```python
from build123d import *
from build123d.topology import SkipClean

# Parameters (mm, degrees)
SKETCH_2_W           = 5
SKETCH_2_H           = 10
EXTRUDE_1_DEPTH      = 0.5
CUT_EXTRUDE_1_DEPTH  = 1.5
EXTRUDE_3_DEPTH      = 0.5
SKETCH_8_R           = 0.6
CUT_EXTRUDE_2_DEPTH  = 0.5
SKETCH_12_W          = 5
SKETCH_12_H          = 0.5
EXTRUDE_4_DEPTH      = 10.5
SKETCH_14_W          = 5
SKETCH_14_H          = 0.5
EXTRUDE_5_DEPTH      = 10
SKETCH_16_W          = 5
SKETCH_16_H          = 0.5
CUT_EXTRUDE_3_DEPTH  = 10
CUT_EXTRUDE_4_DEPTH  = 10
EXTRUDE_START        = -0.5
EXTRUDE_6_DEPTH      = 0.5
SKETCH_19_R          = 0.6
CUT_EXTRUDE_5_DEPTH  = 0.5
SKETCH_23_W          = 0.5
SKETCH_23_H          = 1.5
EXTRUDE_7_DEPTH      = 0.5
EXTRUDE_9_DEPTH      = 0.5
SKETCH_25_R          = 0.25
CUT_EXTRUDE_6_DEPTH  = 0.5
CUT_EXTRUDE_START    = -0.5
SKETCH_28_R          = 0.25
CUT_EXTRUDE_7_DEPTH  = 0.5
SCALE_1_SCALE        = 3.181818182
SCALE_2_SCALE        = 0.771428571
CUT_EXTRUDE_8_DEPTH  = 10
SKETCH_30_R          = 1.75
CUT_EXTRUDE_9_DEPTH  = 10
EXTRUDE_10_DEPTH     = 3
SKETCH_37_R          = 4.295454545
EXTRUDE_11_DEPTH     = 3
CUT_EXTRUDE_START_2  = -3
SKETCH_38_R          = 1.75
CUT_EXTRUDE_10_DEPTH = 3
SKETCH_39_R          = 1.75
CUT_EXTRUDE_11_DEPTH = 3
SKETCH_41_W          = 46.80206249
SKETCH_41_H          = 2.589600393
CUT_EXTRUDE_13_DEPTH = 30.175477213
SKETCH_42_W          = 32.065343688
SKETCH_42_H          = 1.095167369
CUT_EXTRUDE_14_DEPTH = 30.175477212
EXTRUDE_START_2      = 0.77
EXTRUDE_12_DEPTH     = 0.77
CUT_EXTRUDE_15_REACH = 34.524
SKETCH_44_R          = 1.75


with BuildPart() as part:
    # 草图2 → 凸台-拉伸1 (new body)
    with BuildSketch(Plane(origin=(0, 0, 0), x_dir=(1, 0, 0), z_dir=(0, 1, 0))):
        Rectangle(SKETCH_2_W, SKETCH_2_H)
    extrude(amount=EXTRUDE_1_DEPTH)

    # 草图3 → 切除-拉伸1 (cut)
    with BuildSketch(Plane(origin=(0, 0.5, 0), x_dir=(1, 0, 0), z_dir=(0, 1, 0))):
        Polygon((-2.5, 0), (-1, 5), (-4.597388324, 7.155522044), (-6.097388324, 2.155522044), align=None)
    extrude(amount=-CUT_EXTRUDE_1_DEPTH, mode=Mode.SUBTRACT)

    # 草图6 → 凸台-拉伸3 (add)
    with BuildSketch(Plane.XZ):
        with BuildLine():
            Line((-1, -5), (2.5, -5))
            ThreePointArc((2.5, -5), (0.75, -6.75), (-1, -5))
        make_face()
    extrude(amount=-EXTRUDE_3_DEPTH)

    # 草图8 → 切除-拉伸2 (cut)
    with BuildSketch(Plane(origin=(0, 0.5, 0), x_dir=(1, 0, 0), z_dir=(0, 1, 0))):
        with Locations(Location((0.858368729, 4.996789463, 0), (0, 0, 270))):
            Circle(SKETCH_8_R)
    extrude(amount=-CUT_EXTRUDE_2_DEPTH, mode=Mode.SUBTRACT)

    # 草图12 → 凸台-拉伸4 (add)
    with BuildSketch(Plane.XZ):
        with Locations((0, 4.75)):
            Rectangle(SKETCH_12_W, SKETCH_12_H)
    extrude(amount=EXTRUDE_4_DEPTH)

    # 草图14 → 凸台-拉伸5 (add)
    with BuildSketch(Plane(origin=(0, 0, 4.5), x_dir=(-1, 0, 0), z_dir=(0, 0, -1))):
        with Locations((0, -10.25)):
            Rectangle(SKETCH_14_W, SKETCH_14_H)
    extrude(amount=EXTRUDE_5_DEPTH)

    # 草图16 → 切除-拉伸3 (cut)
    with BuildSketch(Plane(origin=(0, -10, 0), x_dir=(1, 0, 0), z_dir=(0, 1, 0))):
        with Locations((0, 5.25)):
            Rectangle(SKETCH_16_W, SKETCH_16_H)
    extrude(amount=-CUT_EXTRUDE_3_DEPTH, mode=Mode.SUBTRACT)

    # 草图17 → 切除-拉伸4 (cut)
    with BuildSketch(Plane(origin=(0, -10, 0), x_dir=(1, 0, 0), z_dir=(0, 1, 0))):
        Polygon((-1, 5), (-2.5, 0), (-4.860653069, 1.950314005), (-3.360653069, 6.950314005), align=None)
    extrude(amount=-CUT_EXTRUDE_4_DEPTH, mode=Mode.SUBTRACT)

    # 草图18 → 凸台-拉伸6 (add)
    with BuildSketch(Plane(origin=(0, -10, 0), x_dir=(1, 0, 0), z_dir=(0, 1, 0)).offset(EXTRUDE_START)):
        with BuildLine():
            Line((-1, 5), (2.5, 5))
            ThreePointArc((2.5, 5), (0.75, 6.75), (-1, 5))
        make_face()
    extrude(amount=EXTRUDE_6_DEPTH)

    # 草图19 → 切除-拉伸5 (cut)
    with BuildSketch(Plane(origin=(0, -10, 0), x_dir=(1, 0, 0), z_dir=(0, 1, 0))):
        with Locations(Location((0.858368729, 4.996789463, 0), (0, 0, 270))):
            Circle(SKETCH_19_R)
    extrude(amount=-CUT_EXTRUDE_5_DEPTH, mode=Mode.SUBTRACT)

    # 草图23 → 凸台-拉伸7 (add)
    with BuildSketch(Plane.XY.offset(5)):
        with Locations((2.25, -0.25)):
            Rectangle(SKETCH_23_W, SKETCH_23_H)
    extrude_7 = extrude(amount=EXTRUDE_7_DEPTH)

    # 草图24 → 凸台-拉伸9 (add)
    with BuildSketch(Plane(origin=(2.5, 0, 0), x_dir=(0, 0, -1), z_dir=(1, 0, 0))):
        with BuildLine():
            Line((-5.5, 0.5), (-5.5, -1))
            ThreePointArc((-5.5, -1), (-6.25, -0.25), (-5.5, 0.5))
        make_face()
    extrude_9 = extrude(amount=-EXTRUDE_9_DEPTH)

    # 草图25 → 切除-拉伸6 (cut)
    with BuildSketch(Plane(origin=(2.5, 0, 0), x_dir=(0, 0, -1), z_dir=(1, 0, 0))):
        with Locations((-5.5, -0.25)):
            Circle(SKETCH_25_R)
    extrude(amount=-CUT_EXTRUDE_6_DEPTH, mode=Mode.SUBTRACT)

    # 镜向1: 凸台-拉伸7, 凸台-拉伸9 across plane
    add(extrude_7.mirror(Plane(origin=(0, 0, 0), x_dir=(0, 0, 1), z_dir=(1, 0, 0))))
    add(extrude_9.mirror(Plane(origin=(0, 0, 0), x_dir=(0, 0, 1), z_dir=(1, 0, 0))))

    # 草图28 → 切除-拉伸7 (cut)
    with BuildSketch(Plane.ZY.offset(2.5).offset(CUT_EXTRUDE_START)):
        with Locations(Location((5.5, -0.25, 0), (0, 0, 180))):
            Circle(SKETCH_28_R)
    extrude(amount=CUT_EXTRUDE_7_DEPTH, mode=Mode.SUBTRACT)


with BuildPart() as part_1:
    # 缩放比例1: scaled about (0.132742616, -4.910605003, 1.535666779)
    add(part.part.scale(SCALE_1_SCALE).moved(Location((-0.289620253, 10.714047279, -3.3505457))))


with BuildPart() as part_2:
    # 缩放比例2: scaled about (0.132742617, -4.910605002, 1.53566678)
    add(part_1.part.scale(SCALE_2_SCALE).moved(Location((0.03034117, -1.122424, 0.35100955))))

    # 草图29 → 切除-拉伸8 (cut)
    with BuildSketch(Plane(origin=(0, 8.369970913, 0), x_dir=(1, 0, 0), z_dir=(0, 1, 0))):
        with BuildLine():
            ThreePointArc((3.397828922, 14.506424406), (1.647828922, 16.256424406), (-0.102171078, 14.506424406))
            Line((-0.102171078, 14.506424406), (0.441118704, 14.506424406))
            ThreePointArc((0.441118704, 14.506424406), (1.913824893, 15.97127127), (3.386531082, 14.506424406))
            Line((3.386531082, 14.506424406), (3.397828922, 14.506424406))
        make_face()
        with BuildLine():
            Line((0.441118704, 14.506424406), (-0.102171078, 14.506424406))
            ThreePointArc((-0.102171078, 14.506424406), (1.647828922, 12.756424406), (3.397828922, 14.506424406))
            Line((3.397828922, 14.506424406), (3.386531082, 14.506424406))
            ThreePointArc((3.386531082, 14.506424406), (3.386546895, 14.502484216), (3.386552166, 14.498543997))
            ThreePointArc((3.386552166, 14.498543997), (1.909884674, 13.025821995), (0.441118704, 14.506424406))
        make_face()
    extrude(amount=-CUT_EXTRUDE_8_DEPTH, mode=Mode.SUBTRACT)

    # 草图30 → 切除-拉伸9 (cut)
    with BuildSketch(Plane(origin=(0, 8.369970913, 0), x_dir=(1, 0, 0), z_dir=(0, 1, 0))):
        with Locations(Location((1.511995488, 4.506424406, 0), (0, 0, 270))):
            Circle(SKETCH_30_R)
    extrude(amount=-CUT_EXTRUDE_9_DEPTH, mode=Mode.SUBTRACT)

    # 草图33 → 凸台-拉伸10 (add)
    with BuildSketch(Plane(origin=(0, 8.369970913, 0), x_dir=(1, 0, 0), z_dir=(0, 1, 0))):
        Polygon((-5.102171078, -10.039030139), (-5.102171078, -11.266302866), (-6.329443805, -11.266302866), (-6.329443805, 2.233697134), (-2.647625624, 14.506424406), (5.943283467, 14.506424406), (5.943283467, -11.266302866), (4.71601074, -11.266302866), (4.71601074, -10.039030139), align=None)
    extrude(amount=EXTRUDE_10_DEPTH)

    # 草图37 → 凸台-拉伸11 (add)
    with BuildSketch(Plane(origin=(0, 8.369970913, 0), x_dir=(1, 0, 0), z_dir=(0, 1, 0))):
        with Locations((1.647828922, 14.506424406)):
            Circle(SKETCH_37_R)
    extrude(amount=EXTRUDE_11_DEPTH)

    # 草图38 → 切除-拉伸10 (cut)
    with SkipClean():  # the faces are left unmerged after this step: merging them gives an invalid solid
        with BuildSketch(Plane(origin=(0, 8.369970913, 0), x_dir=(-1, 0, 0), z_dir=(0, -1, 0)).offset(CUT_EXTRUDE_START_2)):
            with Locations(Location((-1.647828922, 14.506424406, 0), (0, 0, 270))):
                Circle(SKETCH_38_R)
        extrude(amount=CUT_EXTRUDE_10_DEPTH, mode=Mode.SUBTRACT)

    # 草图39 → 切除-拉伸11 (cut)
    with BuildSketch(Plane(origin=(0, 8.369970913, 0), x_dir=(-1, 0, 0), z_dir=(0, -1, 0)).offset(CUT_EXTRUDE_START_2)):
        with Locations(Location((-1.511995488, 4.506424406, 0), (0, 0, 270))):
            Circle(SKETCH_39_R)
    extrude(amount=CUT_EXTRUDE_11_DEPTH, mode=Mode.SUBTRACT)

    # 草图41 → 切除-拉伸13 (cut, through all)
    with BuildSketch(Plane(origin=(5.943283467, 0, 0), x_dir=(0, 0, -1), z_dir=(1, 0, 0))):
        with Locations((1.937836064, 10.437498382)):
            Rectangle(SKETCH_41_W, SKETCH_41_H)
    extrude(amount=-CUT_EXTRUDE_13_DEPTH, mode=Mode.SUBTRACT)

    # 草图42 → 切除-拉伸14 (cut, through all)
    with BuildSketch(Plane(origin=(5.943283467, 0, 0), x_dir=(0, 0, -1), z_dir=(1, 0, 0))):
        with Locations((4.766368978, 8.917554598)):
            Rectangle(SKETCH_42_W, SKETCH_42_H)
    extrude(amount=-CUT_EXTRUDE_14_DEPTH, mode=Mode.SUBTRACT)

    # 草图43 → 凸台-拉伸12 (add)
    with BuildSketch(Plane.XZ.offset(-7.142698186).offset(EXTRUDE_START_2)):
        with BuildLine():
            Line((-6.329443805, 8.811757412), (5.943283467, 8.811757412))
            Line((5.943283467, 8.811757412), (5.943283467, -14.506424406))
            ThreePointArc((5.943283467, -14.506424406), (4.685173959, -17.543769444), (1.647828922, -18.801878952))
            ThreePointArc((1.647828922, -18.801878952), (-1.389516115, -17.543769444), (-2.647625624, -14.506424406))
            Line((-2.647625624, -14.506424406), (-6.329443805, -2.233697134))
            Line((-6.329443805, -2.233697134), (-6.329443805, 8.811757412))
        make_face()
    extrude(amount=-EXTRUDE_12_DEPTH)

    # 草图44 → 切除-拉伸15 (cut, up to next)
    with BuildSketch(Plane(origin=(0, 7.142698186, 0), x_dir=(1, 0, 0), z_dir=(0, 1, 0)), mode=Mode.PRIVATE) as cut_extrude_15_sk1:
        with Locations(Location((1.511995488, 4.506424406, 0), (0, 0, 270))):
            Circle(SKETCH_44_R)
    cut_extrude_15_tool1 = extrude(cut_extrude_15_sk1.sketch, amount=-CUT_EXTRUDE_15_REACH, mode=Mode.PRIVATE) & part_2.part
    # 草图44 → 切除-拉伸15 (cut, up to next)
    with BuildSketch(Plane(origin=(0, 7.142698186, 0), x_dir=(1, 0, 0), z_dir=(0, 1, 0)), mode=Mode.PRIVATE) as cut_extrude_15_sk2:
        with Locations(Location((1.647828922, 14.506424406, 0), (0, 0, 270))):
            Circle(SKETCH_44_R)
    cut_extrude_15_tool2 = extrude(cut_extrude_15_sk2.sketch, amount=-CUT_EXTRUDE_15_REACH, mode=Mode.PRIVATE) & part_2.part
    add(cut_extrude_15_tool1.solids().sort_by_distance((1.511995, 7.142698, -4.506424))[0], mode=Mode.SUBTRACT)
    add(cut_extrude_15_tool2.solids().sort_by_distance((1.647829, 7.142698, -14.506424))[0], mode=Mode.SUBTRACT)


solid = part_2.part
```
Work out the finished part from the listing and answer in its coordinate system (mm). A direction names the side the tool comes from. Give positions to 0.01 mm unless a question says otherwise; leave off trailing zeros. Write each loop counter-clockwise with the first axis right and the second up, starting at its lowest first coordinate (ties: lowest second). Pieces come first, ordered by that corner, then holes. Notation, with made-up numbers: (-25, 27.25) - (31, 27.25) arc R29 ccw to (31, 49.25) - close; hole circle Ø9 at (16, -12). An arc over 180 degrees is marked (long way). Use one line per item in the form item = value.
1. Determine the mould class of faces 5 (the face through (-6.329, -2, 9)), 6 (the face through (0, -18.63, -1)), 7 (the face through (0, 8.37, 0)), 8 (the face through (0, 6.373, -2)) for opening direction Y: released by +Y, released by -Y, zero draft, split by the parting line, or undercut.
Filled in:
face_5 = zero draft
face_6 = released by -Y
face_7 = released by +Y
face_8 = undercut
2. A cutting plane is placed at D-D (x = -3.5). Write down the section's boundary in (y, z).
Filled in:
outline = (-18.63, -11.67) - (-17.4, -11.67) - (-17.4, 8.81) - (6.37, 8.81) - (6.37, -11.67) - (8.37, -11.67) - (8.37, 10.04) - (-18.63, 10.04) - close
3. A cutting plane is placed at C-C (y = -11.25). Write down the section's boundary in (x, z).
Filled in:
outline = (-6.33, 8.81) - (5.94, 8.81) - (5.94, 10.04) - (-6.33, 10.04) - close
4. A cutting plane is placed at B-B (z = -5). Write down the section's boundary in (x, y).
Filled in:
outline = (-5.5, -18.63) - (5.94, -18.63) - (5.94, -17.4) - (-5.5, -17.4) - close; (-5.5, 6.37) - (-0.17, 6.37) - (-0.17, 8.37) - (-5.5, 8.37) - close; (3.19, 6.37) - (5.94, 6.37) - (5.94, 8.37) - (3.19, 8.37) - close
5. For faces 1 (the face through (4.716, 7, 12)), 2 (the face through (-6, 4.688, 11)), 3 (the face through (0, -17.403, -2)), 4 (the face through (0.84, 7.39, -2.89)), determine the directions among +Z, -Z, +X, -X, +Y, -Y from which every point of the face is accessible in a straight line to the end or side of a thin tool.
Filled in:
face_1 = +Z, +Y, -Y
face_2 = +Z, +X, -X, -Y
face_3 = -Z, +X, -X
face_4 = +Y
6. Each of these flat-tipped pins is pushed along its axis until it touches: pin 1 Ø6 at (x, y) = (3, -6) entering from +Z; pin 2 Ø1.1 at (y, z) = (6.53, 11.27) entering from -X; pin 3 Ø3.5 at (x, y) = (-2.5, -4.5) entering from -Z. Where does it stop, or does it pass through?
Filled in:
pin_1 = 10.04
pin_2 = through
pin_3 = 8.81
7. Consider L1, parallel to Y at x = -2.75, z = 5; L2, parallel to Z at x = 0.75, y = 3.25; L3, parallel to Y at x = 4.75, z = 11. Determine where each line is inside the solid, lowest interval first.
Filled in:
L1 = -18.63 to -17.4, 6.37 to 8.37
L2 = 8.81 to 10.04
L3 = 4.69 to 5.98, 7.08 to 8.37
8. A cutting plane is placed at A-A (z = 2). Write down the section's boundary in (x, y), and give its area (3 significant figures).
Filled in:
outline = (-6.33, -18.63) - (5.94, -18.63) - (5.94, -17.4) - (-6.33, -17.4) - close; (-6.33, 6.37) - (5.94, 6.37) - (5.94, 8.37) - (-6.33, 8.37) - close
area = 39.6 mm^2
